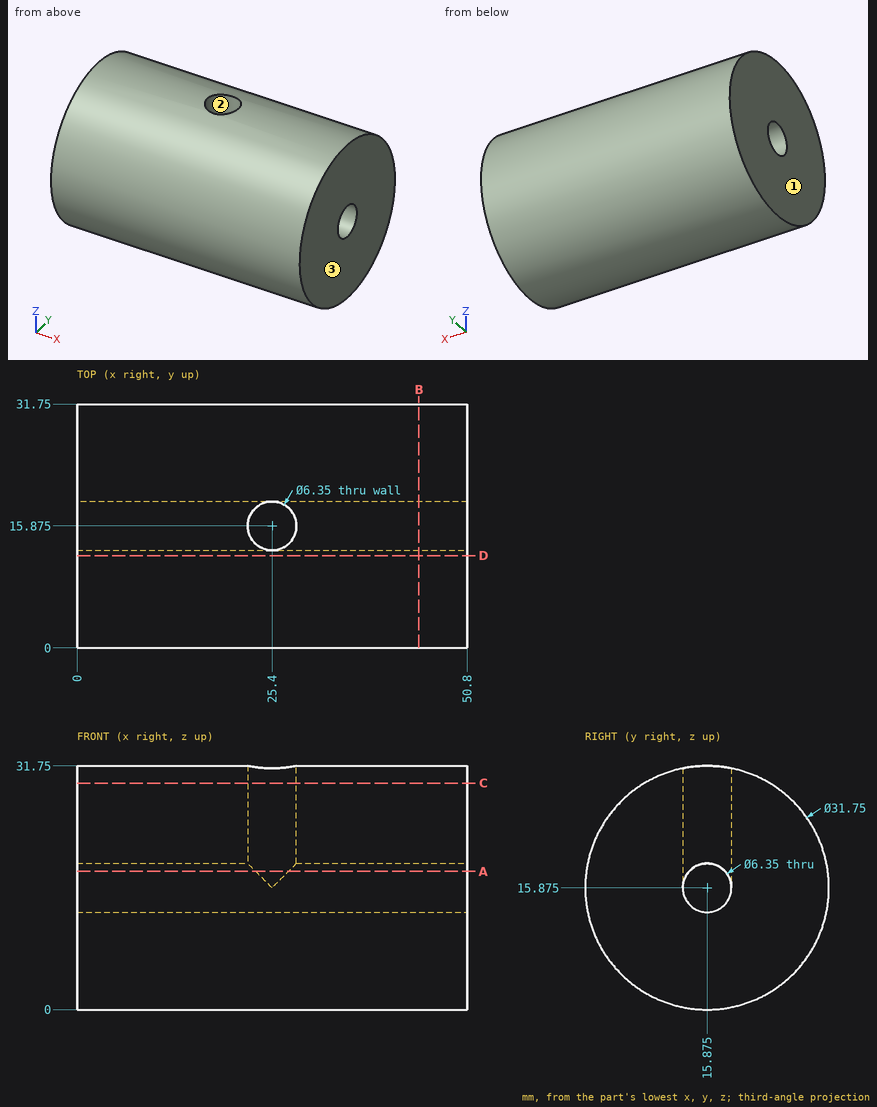
Check sheet for the drawn part. Datum: minimum x, y, z corner. Units: mm. Give positions to 0.01 mm unless a question says otherwise; leave off trailing zeros. Loops run counter-clockwise (first coordinate to the right, second up) from the corner with the lowest first, then second, coordinate; pieces in that order, holes last.
1) Sectioned sample at B-B, the plane x = 44.5. Enter the section's corners in (y, z) (3 decimals).
2) Sectioned sample at A-A, the plane z = 18. Enter the section's corners in (x, y) (3 decimals).
3) Sectioned sample at D-D, the plane y = 12. Enter the section's corners in (x, z), then the cut area to 3 significant figures.
4) Draft check along X on the marked faces 1, 2 and 3. Enter one of: pulls with the +X half, pulls with the -X half, needs draft (parallel to the pull), parting line crosses it, or undercut.
5) Depth check by flat-ended pin: pin 1 Ø6 at (x, z) = (37.5, 21) entering from -Y; pin 2 Ø8 at (x, y) = (24, 23.5) entering from -Z; pin 3 Ø1 at (x, z) = (35, 13.5) entering from +Y; pin 4 Ø5 at (y, z) = (15.875, 15.875) entering from +X. Enter the tip coordinate at first touch or a pass-through.
6) Sectioned sample at C-C, the plane z = 29.5. Enter the section's corners in (x, y) (3 decimals).
7) Thickness scan on line 1 along Y through (x, z) = (19, 16); line 2 along Y through (x, z) = (18, 14); line 3 along Z through (x, y) = (38, 14.5). Record the ranges inside material, lowest first.
Answers:
1. outline: circle Ø31.75 at (15.875, 15.875); hole circle Ø6.35 at (15.875, 15.875)
2. outline: (0, 0.143) - (50.8, 0.143) - (50.8, 13.516) - (27.525, 13.516) arc R3.175 cw to (23.275, 13.516) - (0, 13.516) - close; (0, 18.234) - (23.275, 18.234) arc R3.175 cw to (27.525, 18.234) - (50.8, 18.234) - (50.8, 31.607) - (0, 31.607) - close
3. outline: (0, 0.48) - (50.8, 0.48) - (50.8, 31.27) - (0, 31.27) - close
3. area: 1,560 mm2
4. face 1: pulls with the -X half
4. face 2: undercut
4. face 3: pulls with the +X half
5. pin 1: stops at y = 0.14
5. pin 2: stops at z = 0.42
5. pin 3: stops at y = 31.64
5. pin 4: passes through
6. outline: (0, 7.728) - (50.8, 7.728) - (50.8, 24.022) - (0, 24.022) - close; hole circle Ø6.35 at (25.4, 15.875)
7. line 1: y = 0 to 12.7, 19.05 to 31.75
7. line 2: y = 0.11 to 13.31, 18.44 to 31.64
7. line 3: z = 0.06 to 13.01, 18.74 to 31.69
